Geometry check sheet. Reference: drawing and pictorial views, mm from the part's lowest x, y, z. A direction names the side the tool comes from. Give positions to 0.01 mm unless a question says otherwise; leave off trailing zeros. Loops run counter-clockwise (first coordinate to the right, second up) from the corner with the lowest first, then second, coordinate; pieces in that order, holes last. Notation, with made-up numbers: (69.5, -21.5) -> (127.5, -21.5) arc R16 cw to (127.5, 4.5) -> close; hole circle Ø7 at (-28, -4). An arc over 180 degrees is marked (long way). Answer in a Markdown table with one row per item. Add a question column.
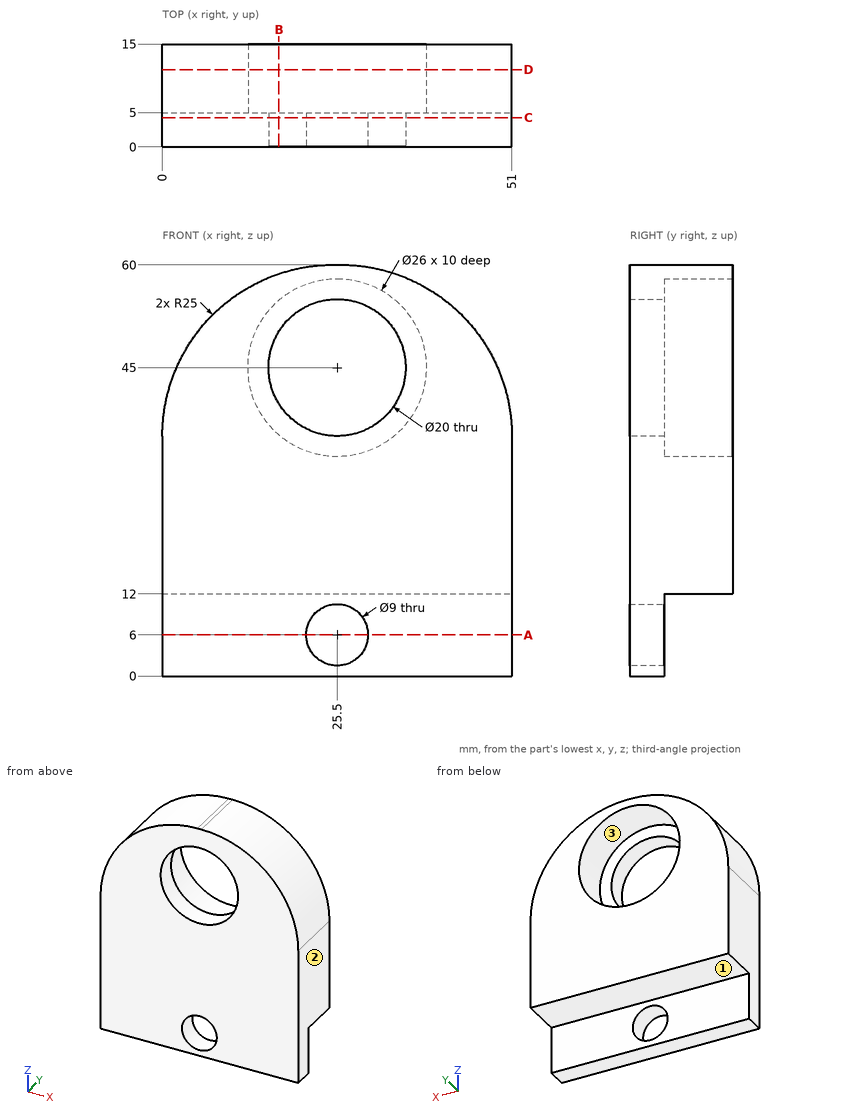
1. Sectioned sample at D-D (y = 11.25). Enter the section's corners in (x, z).
2. Material ranges on L1, parallel to X at y = 3.9, z = 6; L2, parallel to Y at x = 16.5, z = 5; L3, parallel to X at y = 2.55, z = 45, recorded low to high. Write a range as from..to.
3. Sectioned sample at A-A (z = 6). Enter the section's corners in (x, y), plus the area to 3 significant figures.
4. Gauge pin test, flat ends, axial feed: pin 1 Ø8 at (x, z) = (26.5, 43) entering from +Y; pin 2 Ø11.5 at (x, z) = (25.5, 6) entering from +Y; pin 3 Ø2 at (y, z) = (10, 50.5) entering from -X. Record the tip position at first contact, or that the pin passes through.
5. Sectioned sample at C-C (y = 4.25). Enter the section's corners in (x, z).
6. Access from +Z, -Z, +X, -X, +Y, -Y to the whole of each face (thin tool, end or side, straight path). Record for the marked faces 1, 2 and 3.
7. Sectioned sample at B-B (x = 17). Enter the section's corners in (y, z).
Response:
| question | item | result |
|---|---|---|
| 1 | outline | (0, 12) -> (51, 12) -> (51, 35) arc R25 ccw to (26, 60) -> (25, 60) arc R25 ccw to (0, 35) -> close; hole circle Ø26 at (25.5, 45) |
| 2 | L1 | x = 0..21, 30..51 |
| 2 | L2 | y = 0..5 |
| 2 | L3 | x = 2.09..15.5, 35.5..48.91 |
| 3 | outline | (0, 0) -> (21, 0) -> (21, 5) -> (0, 5) -> close; (30, 0) -> (51, 0) -> (51, 5) -> (30, 5) -> close |
| 3 | area | 210 mm2 |
| 4 | pin 1 | passes through |
| 4 | pin 2 | stops at y = 5 |
| 4 | pin 3 | stops at x = 4.63 |
| 5 | outline | (0, 0) -> (51, 0) -> (51, 35) arc R25 ccw to (26, 60) -> (25, 60) arc R25 ccw to (0, 35) -> close; hole circle Ø20 at (25.5, 45); hole circle Ø9 at (25.5, 6) |
| 6 | face 1 | -Z, +X, -X, +Y |
| 6 | face 2 | +Z, -Z, +X, +Y, -Y |
| 6 | face 3 | +Y |
| 7 | outline | (0, 0) -> (5, 0) -> (5, 12) -> (15, 12) -> (15, 35.16) -> (5, 35.16) -> (5, 39.73) -> (0, 39.73) -> close; (0, 50.27) -> (5, 50.27) -> (5, 54.84) -> (15, 54.84) -> (15, 58.69) -> (0, 58.69) -> close |
